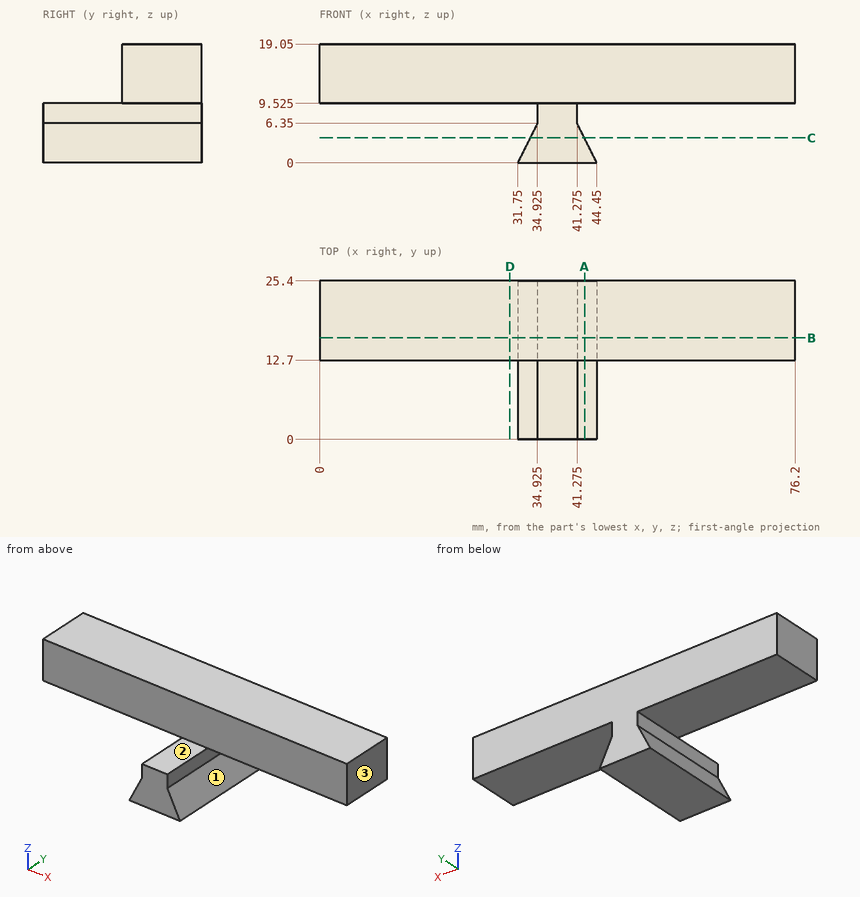
Can you work these out from the drawing? Everything is in mm from the part's minimum corner. A direction names the side the tool comes from. Round coordinates to 2 decimals unless told otherwise and drop trailing zeros. Write each loop counter-clockwise with the first axis right and the second up, starting at its lowest first coordinate (ties: lowest second). Pieces come first, ordered by that corner, then holes. Notation, with made-up numbers: (89, 17) - (118, 17) arc R26 ccw to (118, 40) - close; hole circle Ø1 at (-8.5, 64.5). An arc over 180 degrees is marked (long way). Write each question's results on one line, items separated by ' | '. Start each with the question number.
1) Which directions (+Z, -Z, +X, -X, +Y, -Y) give clear straight access to the entire face, cutting with the end or side of a thin tool? Please do the marked faces 1, 2 and 3.
2) For pin 1 Ø10 at (x, y) = (9.5, 13.5) entering from -Z (3 decimals); pin 2 Ø1.6 at (y, z) = (10, 8) entering from -X (3 decimals); pin 3 Ø3 at (x, z) = (29, 14) entering from -Y, each with a flat end and sliding along its axis, tell me the tip position at first contact or that it passes through.
3) Suppose I cut it at C-C (z = 4). List the corners of the cut face in (x, y) for me.
4) Suppose I cut it at D-D (x = 30.5). List the corners of the cut face in (y, z) for me (3 decimals).
5) Please list where these lines run through material, in increasing order: line 1 (Z direction, x = 51, y = 13) (3 decimals); line 2 (X direction, y = 21.5, z = 8.5) (3 decimals); line 3 (Y direction, x = 15, z = 17.5).
6) Suppose I cut it at B-B (y = 16.25). List the corners of the cut face in (x, z) for me (3 decimals), and give its area (3 significant figures).
7) Suppose I cut it at A-A (x = 42.5). List the corners of the cut face in (y, z) for me (3 decimals).
Here are the results:
1) face 1: +X, +Y, -Y | face 2: +Z, +X, -X, -Y | face 3: +Z, -Z, +X, +Y, -Y
2) pin 1: stops at z = 9.525 | pin 2: stops at x = 34.925 | pin 3: stops at y = 12.7
3) outline: (33.75, 0) - (42.45, 0) - (42.45, 25.4) - (33.75, 25.4) - close
4) outline: (12.7, 9.525) - (25.4, 9.525) - (25.4, 19.05) - (12.7, 19.05) - close
5) line 1: z = 9.525 to 19.05 | line 2: x = 34.925 to 41.275 | line 3: y = 12.7 to 25.4
6) outline: (0, 9.525) - (34.925, 9.525) - (34.925, 6.35) - (31.75, 0) - (44.45, 0) - (41.275, 6.35) - (41.275, 9.525) - (76.2, 9.525) - (76.2, 19.05) - (0, 19.05) - close | area: 806 mm2
7) outline: (0, 0) - (25.4, 0) - (25.4, 3.9) - (0, 3.9) - close; (12.7, 9.525) - (25.4, 9.525) - (25.4, 19.05) - (12.7, 19.05) - close
